```python
from build123d import *

# Parameters (mm, degrees)
F1_DEPTH    = 25.4
F2_T1_DEPTH = 187.96
F2_T3_DEPTH = 212.2513193251
F3_SIZE     = 12.7
F5_D        = 6.35
F6_D        = 6.35
F6_DEPTH    = 12.7
F6_TIP      = 1.9077324654


# Not quite as in the source:
# - a fillet or chamfer that OpenCascade refuses, or shapes differently, is made with other operations: its cross-section is extruded or revolved along the edge and cut away or added


with BuildPart() as f1:
    # F0 (on Front) → F1 (new body)
    with BuildSketch(Plane.XZ):
        Polygon((-98.3372926712, 35.933367908), (-93.2035595179, 35.933367908), (-93.2035595179, 95.180105418), (-146.8319296837, 95.180105418), (-146.8319296837, 30.8260507882), (-98.3372926712, 30.8260507882), align=None)
    extrude(amount=F1_DEPTH)

    # F2: fillet of radius 32.512 on 2 edges, made by hand

    # F2_s2 → F2_t1 (cut)
    with BuildSketch(Plane.XZ.offset(-81.28)):
        with BuildLine():
            ThreePointArc((-93.2035595179, 62.668105418), (-102.7261038479, 85.6575610879), (-125.7155595179, 95.180105418))
            Line((-125.7155595179, 95.180105418), (-93.2035595179, 95.180105418))
            Line((-93.2035595179, 95.180105418), (-93.2035595179, 62.668105418))
        make_face()
    extrude(amount=F2_T1_DEPTH, mode=Mode.SUBTRACT)

    # F2_s4 → F2_t3 (cut)
    with BuildSketch(Plane.YZ.offset(-226.1434042633)):
        with BuildLine():
            ThreePointArc((0, 95.180105418), (-18.2676718655, 83.7755155861), (-25.4, 63.4555155861))
            Line((-25.4, 63.4555155861), (-25.4, 95.180105418))
            Line((-25.4, 95.180105418), (0, 95.180105418))
        make_face()
    extrude(amount=F2_T3_DEPTH, mode=Mode.SUBTRACT)

    # F3
    f3_edges = [f1.edges().sort_by_distance(p)[0] for p in [
        (-122.584611, 0, 30.826051),
        (-146.83193, -12.7, 30.826051),
    ]]
    chamfer(f3_edges, length=F3_SIZE)

    # F5 (through all)
    with Locations(Plane.XZ.offset(25.4)):
        with Locations((-103.0430421233, 58.3359822631)):
            Hole(F5_D / 2)

    # F6
    with Locations(Plane.XZ.offset(25.4)):
        with Locations((-131.3667148352, 54.4626787305), (-107.1459278464, 42.1714857221), (-129.1075199842, 36.9423851371)):
            Hole(F6_D / 2, depth=F6_DEPTH)
            with Locations((0, 0, -(F6_DEPTH + F6_TIP / 2))):  # 118° drill point
                Cone(0, F6_D / 2, F6_TIP, mode=Mode.SUBTRACT)


solid = f1.part
```
For this review, take the finished solid that the model builds, in its own axes (mm). A direction names the side the tool comes from. Coordinates: 2 decimals unless noted, no trailing zeros. Loops run counter-clockwise (first coordinate to the right, second up) from the corner with the lowest first, then second, coordinate; pieces in that order, holes last. Notation, with made-up numbers: (63, -6) - (101, -6) arc R12 cw to (101, 16) - close; hole circle Ø7 at (49, 19.5). An arc over 180 degrees is marked (long way). Use one line per item in the form item = value. Start each with the question number.
1) Draft analysis for pull direction X (two halves, no side actions). For faces 1 (the face through (-132.04, -18.96, 35.73)), 2 (the face through (-98.337, -18, 33)), 3 (the face through (-120, 0, 70)), 4 (the face through (-146.832, -13, 64)), state which applies: released by +X, released by -X, zero draft, split by the parting line, or undercut.
2) To check wall thickness, follow probe 1 along X at (y, z) = (-10, 58); probe 2 along Y at (x, z) = (-132.5, 64.5); probe 3 along Z at (x, y) = (-136, -16). State the ranges of each line that lie inside material, in increasing order. Write a range as from..to.
3) Take a section at C-C (x = -112.5). State the section outline as (y, z) points.
4) Take a section at D-D (z = 71.5). State the section outline as (x, y) points, plus the area to 3 significant figures.
5) Take a section at A-A (y = -5.5). State the section outline as (x, z) points (3 decimals), plus the area to 3 significant figures.
6) For faces 5 (the face through (-134.3, -18.96, 53.25)), 6 (the face through (-126.355, -18.074, 84.014)), 7 (the face through (-96, -16, 35.933)), list the 3-axis set-ups (+Z, -Z, +X, -X, +Y, -Y) from which the entire face can be reached by the end or side of a thin tool; tool diameter is ignored.
7) For pin 1 (8 mm diameter, centred on x = -119, y = -5, fed in from +Z); pin 2 (1.5 mm diameter, centred on x = -127.5, y = -7.5, fed in from +Z); pin 3 (5 mm diameter, centred on x = -103.04, z = 58.34, fed in from -Y); pin 4 (1.5 mm diameter, centred on y = -18, z = 32.5, fed in from +X), all flat-tipped, find the tip position at first contact; note any pin that passes through.
8) Take a section at B-B (y = -17.5). State the section outline as (x, z) points (3 decimals).
From the geometry:
q1.face_1 = undercut
q1.face_2 = released by +X
q1.face_3 = zero draft
q1.face_4 = released by -X
q2.probe_1 = -146.83..-106.2, -99.89..-93.2
q2.probe_2 = -25.38..0
q2.probe_3 = 32.69..86.32
q3.outline = (-25.4, 30.83) - (-12.7, 30.83) - (0, 43.53) - (0, 92.37) - (-7.75, 92.37) arc R32.51 ccw to (-25.4, 63.46) - close
q4.outline = (-146.83, -24.39) - (-94.43, -24.39) - (-94.43, 0) - (-146.83, 0) - close
q4.area = 1,280 mm2
q5.outline = (-146.832, 43.526) - (-141.332, 38.026) - (-93.204, 38.026) - (-93.204, 62.668) arc R32.512 ccw to (-115.168, 93.422) - (-146.832, 93.422) - close; hole circle Ø6.35 at (-103.043, 58.336)
q5.area = 2,740 mm2
q6.face_5 = -Y
q6.face_6 = +Z, +X, -X, -Y
q6.face_7 = -Z, +X, +Y, -Y
q7.pin_1 = 94.82
q7.pin_2 = 92.86
q7.pin_3 = through
q7.pin_4 = -98.34
q8.outline = (-146.832, 43.526) - (-134.132, 30.826) - (-98.337, 30.826) - (-98.337, 35.933) - (-93.204, 35.933) - (-93.204, 62.668) arc R32.512 ccw to (-101.806, 84.699) - (-146.832, 84.699) - close; hole circle Ø6.35 at (-131.367, 54.463); hole circle Ø6.35 at (-129.108, 36.942); hole circle Ø6.35 at (-107.146, 42.171); hole circle Ø6.35 at (-103.043, 58.336)
